Design review of the part shown in the three views and the two pictorial views. Dimensions are in mm from the part's minimum x, y and z. A direction names the side the tool comes from. Coordinates: 2 decimals unless noted, no trailing zeros. Loops run counter-clockwise (first coordinate to the right, second up) from the corner with the lowest first, then second, coordinate; pieces in that order, holes last. Notation, with made-up numbers: (31.5, -39.5) -> (72.5, -39.5) arc R6 cw to (72.5, -29.5) -> close; hole circle Ø3 at (57, 24). An arc over 180 degrees is marked (long way). Answer in a Markdown table with one row per item.
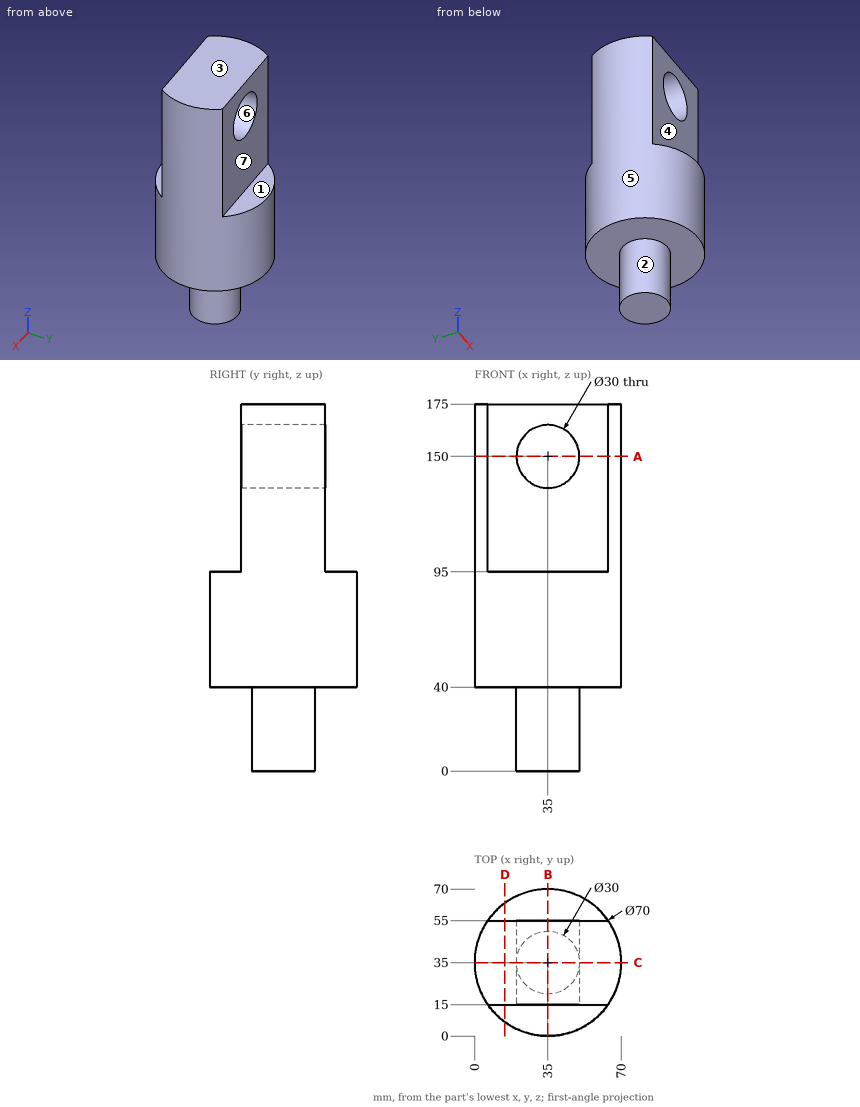
Item 1: Insertion check: pin 1 (3 mm diameter, centred on y = 38, z = 138, fed in from -X); pin 2 (17 mm diameter, centred on x = 26, z = 148.5, fed in from -Y); pin 3 (2 mm diameter, centred on x = 9.5, y = 10.5, fed in from -Z); pin 4 (12 mm diameter, centred on x = 41.5, y = 60, fed in from +Z). Each pin has a flat end and moves straight along its axis. Give the tip position at first contact, or say it passes through.
Worked answers:
| item | result |
|---|---|
| pin 1 | x = 0.03 |
| pin 2 | y = 15 |
| pin 3 | z = 40 |
| pin 4 | z = 175 |
Item 2: The part is to be moulded in two halves that separate along X. For the marked faces 5, 6 and 7, say which applies: +X half, -X half, draft (parallel to the pull), parting line (faces both ways), or undercut.
Worked answers:
| item | result |
|---|---|
| face 5 | parting line |
| face 6 | undercut |
| face 7 | draft |
Item 3: For the marked faces 1, 2, 3 and 4, list the 3-axis set-ups (+Z, -Z, +X, -X, +Y, -Y) from which the entire face can be reached by the end or side of a thin tool; tool diameter is ignored.
Worked answers:
| item | result |
|---|---|
| face 1 | +Z, +X, -X, +Y |
| face 2 | -Z |
| face 3 | +Z, +X, -X, +Y, -Y |
| face 4 | +Z, +X, -X, -Y |
Item 4: For L1, parallel to X at y = 36.5, z = 151; L2, parallel to Z at x = 23.5, y = 56; L3, parallel to X at y = 37, z = 150, list the stretches that pass through material, from the lowest coordinate up.
Worked answers:
| item | result |
|---|---|
| L1 | 0.03 to 20.03, 49.97 to 69.97 |
| L2 | 40 to 95 |
| L3 | 0.06 to 20, 50 to 69.94 |
Item 5: Take a section at C-C, the plane y = 35. State the section outline as (x, z) points, and give its area (3 significant figures).
Worked answers:
| item | result |
|---|---|
| outline | (0, 40) -> (20, 40) -> (20, 0) -> (50, 0) -> (50, 40) -> (70, 40) -> (70, 175) -> (0, 175) -> close; hole circle Ø30 at (35, 150) |
| area | 9,940 mm² |
Item 6: Take a section at D-D, the plane x = 14.5. State the section outline as (y, z) points.
Worked answers:
| item | result |
|---|---|
| outline | (6.63, 40) -> (63.37, 40) -> (63.37, 95) -> (55, 95) -> (55, 175) -> (15, 175) -> (15, 95) -> (6.63, 95) -> close |
Item 7: Take a section at A-A, the plane z = 150. State the section outline as (x, y) points, and give its area (3 significant figures).
Worked answers:
| item | result |
|---|---|
| outline | (6.28, 15) -> (20, 15) -> (20, 55) -> (6.28, 55) arc R35 ccw to start; (50, 15) -> (63.72, 15) arc R35 ccw to (63.72, 55) -> (50, 55) -> close |
| area | 1,440 mm² |
Item 8: Take a section at B-B, the plane x = 35. State the section outline as (y, z) points, and give its area (3 significant figures).
Worked answers:
| item | result |
|---|---|
| outline | (0, 40) -> (20, 40) -> (20, 0) -> (50, 0) -> (50, 40) -> (70, 40) -> (70, 95) -> (55, 95) -> (55, 135) -> (15, 135) -> (15, 95) -> (0, 95) -> close; (15, 165) -> (55, 165) -> (55, 175) -> (15, 175) -> close |
| area | 7,050 mm² |
